Input: dimensioned drawing with shaded views. Units: mm. Origin: part minimum x, y, z. A direction names the side the tool comes from. Coordinates: 2 decimals unless noted, no trailing zeros. Write item = value, one per line. Start each with the question number.
Item 1: Set-up query: the marked faces 1 and 2. Return all of +Z, -Z, +X, -X, +Y, -Y with unobstructed straight access to the full face (end or side cutting, diameter ignored); none if empty.
Item 2: Mould query, pull axis X, two halves, no side actions, for the marked faces 3, 4, 5 and 6. Classes: released by +X, released by -X, zero draft, split by the parting line, or undercut.
Item 3: Contact query for flat-ended pins moving along their axis: pin 1 (6 mm diameter, centred on x = 23, y = 6, fed in from -Z); pin 2 (12 mm diameter, centred on x = 11.5, y = 21.5, fed in from -Z). Output: stop coordinate, or through.
Item 4: Ray query, line 1 along X through (y, z) = (1.5, 40). Return the intervals inside material, ascending. Write a range as [from, to].
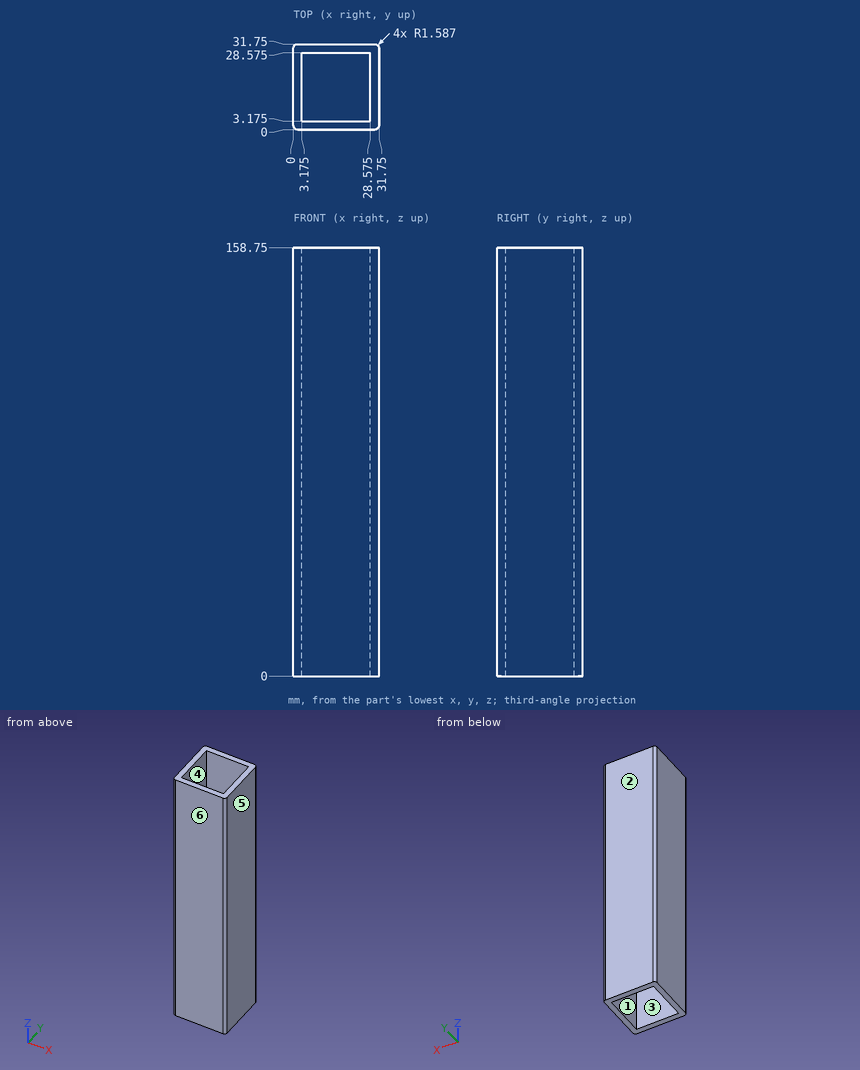
Computed:
q1.face_1 = +Z, -Z
q1.face_2 = +Z, -Z, +X, -X, +Y
q2.face_3 = undercut
q2.face_4 = undercut
q2.face_5 = released by +X
q2.face_6 = zero draft
q3.pin_1 = 0
q3.pin_2 = through
q4.line_1 = [0, 31.75]
